Read the model definition and answer for the solid it produces. Units are mm, in the model's axes. Face numbers are marked on the shaded views. A direction names the side the tool comes from. Give positions to 0.01 mm unless a question says otherwise; leave off trailing zeros. Loops run counter-clockwise (first coordinate to the right, second up) from the corner with the lowest first, then second, coordinate; pieces in that order, holes last. Notation, with made-up numbers: M -30.75,44 L 21.25,44 A21 cw 21.25,69 Z; hole C -19.5,89.5 d2. An arc over 180 degrees is marked long. Return JSON: item names as keys, results as strings. Group by question number.
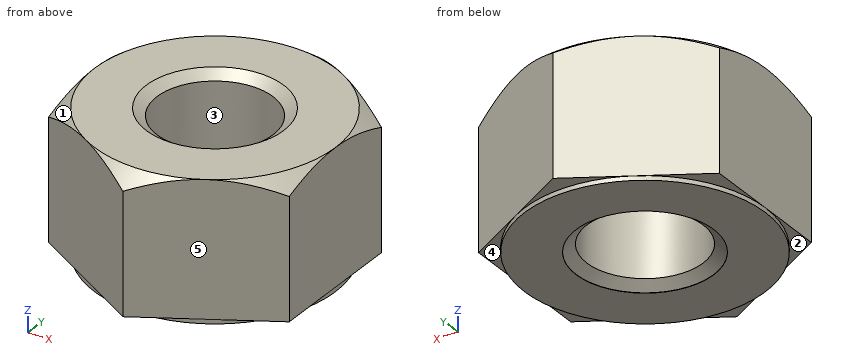
```python
from build123d import *

# Parameters (mm, degrees)
BASENUT_START = -12.8016
BASENUTSKE_R  = 5.35813
BASENUT_DEPTH = 12.8016
SKETCH4_W     = 0.4064
SKETCH4_H     = 14.419109733


with BuildPart() as part:
    # BaseNutSke → BaseNut (new body)
    with BuildSketch(Plane.XY.offset(BASENUT_START)):
        Polygon((11.1125, 6.415804866), (11.1125, -6.415804866), (0, -12.831609733), (-11.1125, -6.415804866), (-11.1125, 6.415804866), (0, 12.831609733), align=None)
        Circle(BASENUTSKE_R, mode=Mode.SUBTRACT)
    extrude(amount=BASENUT_DEPTH)

    # Sketch4 → Bearing-Face (revolve, cut)
    with BuildSketch(Plane(origin=(0, 0, 0), x_dir=(0, 0, -1), z_dir=(1, 0, 0)), mode=Mode.PRIVATE) as bearing_face_sk:
        with Locations((12.5984, 18.322054867)):
            Rectangle(SKETCH4_W, SKETCH4_H)
        Polygon((0, 11.1125), (-12.7, 11.1125), (-12.7, 25.531609733), (1.27, 25.531609733), (1.27, 12.831609733), align=None)
    revolve(bearing_face_sk.sketch.rotate(Axis((0, 0, 0), (0, 0, -1)), 270), axis=Axis((0, 0, 0), (0, 0, -1)), mode=Mode.SUBTRACT)

    # Sketch5 → EndChamfer (revolve, cut)
    with BuildSketch(Plane(origin=(0, 0, 0), x_dir=(0, 0, -1), z_dir=(1, 0, 0)), mode=Mode.PRIVATE) as endchamfer_sk:
        Polygon((12.7762, 6.35), (12.012233664, 5.258943), (12.827, 5.258943), (12.827, 6.35), align=None)
        Polygon((-0.0508, 6.35), (0, 6.35), (0.763966336, 5.258943), (-0.0508, 5.258943), align=None)
    revolve(endchamfer_sk.sketch.rotate(Axis((0, 0, -25.037505729), (0, 0, -1)), 90), axis=Axis((0, 0, -25.037505729), (0, 0, -1)), mode=Mode.SUBTRACT)


solid = part.part
```
1. Straight lines are drawn through the part: line 1 along Y through (x, z) = (0, -12.75); line 2 along X through (y, z) = (-3, -4.5); line 3 along Y through (x, z) = (-7.25, -7). For each, find the intervals that lie inside material, in ascending order.
2. The mould has two halves that part along Y. Classify the marked faces 3, 4 and 5: +Y half, -Y half, draft (parallel to the pull), parting line (faces both ways), or undercut.
3. Flat-ended cylindrical pins translate along their axes: P1, Ø12.5, axis at x = 0, y = 0, coming from the +Z side; P2, Ø3, axis at x = -3.5, y = 3, coming from the -Z side. Find the tip coordinate at first contact, or state that the pin passes through.
4. For the marked faces 1 and 2, determine the directions among +Z, -Z, +X, -X, +Y, -Y from which every point of the face is accessible in a straight line to the end or side of a thin tool.
5. Find section A-A (z = -1.75). Write down the section's boundary in (x, y).
Result:
{
 "1": {"line 1": "y = -11.11 to -6.31, 6.31 to 11.11", "line 2": "x = -11.11 to -4.44, 4.44 to 11.11", "line 3": "y = -8.65 to 8.65"},
 "2": {"face 3": "undercut", "face 4": "draft", "face 5": "-Y half"},
 "3": {"P1": "stops at z = -0.07", "P2": "stops at z = -12.61"},
 "4": {"face 1": "+Z, -X, -Y", "face 2": "-Z, -X, -Y"},
 "5": {"outline": "M -11.11,-6.42 L 0,-12.83 L 11.11,-6.42 L 11.11,6.42 L 0,12.83 L -11.11,6.42 Z; hole C 0,0 d10.72"}
}
